Source: CAD feature listing. Evaluate the final solid. Frame: model axes, mm. A direction names the side the tool comes from. Give positions to 0.01 mm unless a question says otherwise; leave off trailing zeros. Order: outer loops, then holes, each group sorted by start corner. A loop starts at its lowest first (then second) coordinate and runs counter-clockwise, first axis right, second up.
```python
from build123d import *

# Parameters (mm, degrees)
SKETCH003_R  = 1.5
PAD_DEPTH    = 50
PAD001_DEPTH = 15


with BuildPart() as bearingmountcutout:
    # Sketch007 → Revolution003 (revolve)
    with BuildSketch(Plane.XZ):
        Polygon((-35, 0), (-35, 4), (-10, 4), (-10, 1.5), (0, 1.5), (0, 0), align=None)
    revolve(axis=Axis((0, 0, 0), (1, 0, 0)))


with BuildPart() as cutouts:
    # Sketch003 → Pad (new body)
    with BuildSketch(Plane.XY):
        with Locations((-22, 5)):
            Circle(SKETCH003_R)
        with Locations((-12, 5)):
            Circle(SKETCH003_R)
        with Locations((-22, -5)):
            Circle(SKETCH003_R)
        with Locations((-12, -5)):
            Circle(SKETCH003_R)
    extrude(amount=-PAD_DEPTH)

    # Fusion001: union BearingMountCutout
    add(bearingmountcutout.part)


with BuildPart() as innerrace002:
    # Sketch001 → Revolution001 (revolve)
    with BuildSketch(Plane.XZ):
        Polygon((-7.853732, 6.200251), (-2.853732, 6.200251), (0, 3.346519), (0, 0), (-7.853732, 0), align=None)
    revolve(axis=Axis((0, 0, 0), (1, 0, 0)))


with BuildPart() as base001:
    # Sketch004 → Pad001 (new body, symmetric)
    with BuildSketch(Plane.XZ):
        Polygon((-26, -20.927391), (-26, 5.975582), (-14.9603, 14.10621), (-4.966401, 14.10621), (-10.240184, -20.927391), align=None)
    extrude(amount=PAD001_DEPTH, both=True)

    # Fusion: union InnerRace002
    add(innerrace002.part)

    # Cut001: cut Cutouts
    add(cutouts.part, mode=Mode.SUBTRACT)


solid = base001.part
```
1) Material intervals for L1, parallel to Y at x = -22, z = -6; L2, parallel to Y at x = -14.25, z = 0; L3, parallel to X at y = 5, z = -5.5, sorted ascending.
Report:
L1: y = -15 to -6.5, -3.5 to 3.5, 6.5 to 15
L2: y = -15 to -4, 4 to 15
L3: x = -26 to -23.5, -20.5 to -13.5, -10.5 to -7.92
2) Section query A-A, the plane y = 0. Return the cut outline in (x, z), and give its area (3 significant figures).
Report:
outline: (-26, -20.93) - (-10.24, -20.93) - (-7.85, -5.07) - (-7.85, -6.2) - (-2.85, -6.2) - (0, -3.35) - (0, -1.5) - (-10, -1.5) - (-10, -4) - (-26, -4) - close; (-26, 4) - (-10, 4) - (-10, 1.5) - (0, 1.5) - (0, 3.35) - (-2.85, 6.2) - (-6.16, 6.2) - (-4.97, 14.11) - (-14.96, 14.11) - (-26, 5.98) - close
area: 521 mm2
3) Draft query along Y for faces 1 (the flat face through (-15, 15, -3)), 2 (the flat face through (-20.56, -0.21, 9.98)), 3 (the flat face through (-15, -15, -3)), 4 (the flat face through (-12, -5, 0)). Return one class per face: +Y half, -Y half, draft (parallel to the pull), parting line (faces both ways), or undercut.
Report:
face 1: +Y half
face 2: draft
face 3: -Y half
face 4: undercut
4) Pin query (flat end, axial travel): pin 1 (2 mm diameter, centred on x = -10, y = 7.5, fed in from -Z); pin 2 (3.5 mm diameter, centred on y = 0, z = 0, fed in from -X); pin 3 (1 mm diameter, centred on y = 5, z = 10, fed in from -X); pin 4 (1.3 mm diameter, centred on x = -11.5, y = 5.5, fed in from -Z). Return the tip coordinate at first contact, or that it passes through.
Report:
pin 1: stops at z = -20.93
pin 2: stops at x = -10
pin 3: stops at x = -21.21
pin 4: stops at z = 0
5) Section query B-B, the plane x = -12. Return the cut outline in (y, z), and give its area (3 significant figures).
Report:
outline: (-15, -20.93) - (-6.5, -20.93) - (-6.5, 0) - (-4, 0) arc R4 cw to (4, 0) - (6.5, 0) - (6.5, -20.93) - (15, -20.93) - (15, 14.11) - (-15, 14.11) - close; (-3.5, -20.93) - (3.5, -20.93) - (3.5, -1.94) arc R4 cw to (-3.5, -1.94) - close
area: 876 mm2
6) Section query C-C, the plane z = -18. Return the cut outline in (x, y).
Report:
outline: (-26, -15) - (-9.8, -15) - (-9.8, 15) - (-26, 15) - close; hole circle Ø3 at (-22, -5); hole circle Ø3 at (-22, 5); hole circle Ø3 at (-12, -5); hole circle Ø3 at (-12, 5)
7) Section query D-D, the plane y = -9. Return the cut outline in (x, z), and give its area (3 significant figures).
Report:
outline: (-26, -20.93) - (-10.24, -20.93) - (-4.97, 14.11) - (-14.96, 14.11) - (-26, 5.98) - close
area: 600 mm2
8) Reachability of faces 5 (the flat face through (-22, -5, 0)), 6 (the flat face through (-10, 0, 14.106)), 7 (the cylindrical face through (-17.888, 1.532, 3.695)) from +Z, -Z, +X, -X, +Y, -Y: full face, straight path, thin tool, end or side. Return the list, or none.
Report:
face 5: -Z
face 6: +Z, +X, -X, +Y, -Y
face 7: -X
